```python
from build123d import *

# Parameters (mm, degrees)
SKETCH1_W           = 15
SKETCH1_H           = 15
SKETCH1_W_2         = 11
SKETCH1_H_2         = 11
BOSS_EXTRUDE1_DEPTH = 140
SKETCH2_R           = 1.6
CUT_EXTRUDE1_DEPTH  = 142.598022585
SKETCH3_R           = 1.6
CUT_EXTRUDE2_DEPTH  = 142.598022585


with BuildPart() as part:
    # Sketch1 → Boss-Extrude1 (new body)
    with BuildSketch(Plane(origin=(0, 0, 0), x_dir=(1, 0, 0), z_dir=(0, 1, 0))):
        with Locations((7.5, 7.5)):
            Rectangle(SKETCH1_W, SKETCH1_H)
        with Locations((7.5, 7.5)):
            Rectangle(SKETCH1_W_2, SKETCH1_H_2, mode=Mode.SUBTRACT)
    extrude(amount=BOSS_EXTRUDE1_DEPTH)

    # Sketch2 → Cut-Extrude1 (cut, through all)
    with BuildSketch(Plane(origin=(15, 0, 0), x_dir=(0, 0, -1), z_dir=(1, 0, 0))):
        with Locations((7.5, 13)):
            Circle(SKETCH2_R)
        with Locations((7.5, 37)):
            Circle(SKETCH2_R)
        with Locations((7.5, 103)):
            Circle(SKETCH2_R)
        with Locations((7.5, 127)):
            Circle(SKETCH2_R)
    extrude(amount=-CUT_EXTRUDE1_DEPTH, mode=Mode.SUBTRACT)

    # Sketch3 → Cut-Extrude2 (cut, through all)
    with BuildSketch(Plane.XY):
        with Locations((7.5, 85)):
            Circle(SKETCH3_R)
        with Locations((7.5, 55)):
            Circle(SKETCH3_R)
    extrude(amount=-CUT_EXTRUDE2_DEPTH, mode=Mode.SUBTRACT)


solid = part.part
```
Verification items for the finished model (mm, model axes). A direction names the side the tool comes from. Coordinates: 2 decimals unless noted, no trailing zeros. Loops run counter-clockwise (first coordinate to the right, second up) from the corner with the lowest first, then second, coordinate; pieces in that order, holes last. Notation, with made-up numbers: (30, 2) -> (44, 2) arc R26 ccw to (44, 25) -> close; hole circle Ø4 at (49.5, 73). An arc over 180 degrees is marked (long way). Answer in a Markdown table with one row per item. Add a question column.
1. Material ranges on probe 1 along Y at (x, z) = (7.5, -14.6); probe 2 along Y at (x, z) = (1.45, -7.5); probe 3 along X at (y, z) = (43, -4.25), recorded low to high. Write a range as [from, to].
2. Section check D-D, the plane y = 20. Enter the section's corners in (x, z).
3. Access from +Z, -Z, +X, -X, +Y, -Y to the whole of each face (thin tool, end or side, straight path). Record for faces 1 (the face through (13, 69, -7)), 2 (the face through (14, 0, -8)).
4. Section check B-B, the plane z = -11. Enter the section's corners in (x, y).
5. Draft check along X on faces 3 (the face through (14.01, 35.58, -8.24)), 4 (the face through (0, 69, -7)), 5 (the face through (5.9, 55.07, -0.99)), 6 (the face through (7.292, 86.586, -0.986)). Enter one of: +X half, -X half, draft (parallel to the pull), parting line (faces both ways), or undercut.
6. Section check A-A, the plane y = 103. Enter the section's corners in (x, z), then the cut area to 3 significant figures.
7. Section check C-C, the plane x = 7.5. Enter the section's corners in (y, z).
Derived:
| question | item | result |
|---|---|---|
| 1 | probe 1 | y = [0, 53.4], [56.6, 83.4], [86.6, 140] |
| 1 | probe 2 | y = [0, 11.4], [14.6, 35.4], [38.6, 101.4], [104.6, 125.4], [128.6, 140] |
| 1 | probe 3 | x = [0, 2], [13, 15] |
| 2 | outline | (0, -15) -> (15, -15) -> (15, 0) -> (0, 0) -> close; hole (2, -13) -> (13, -13) -> (13, -2) -> (2, -2) -> close |
| 3 | face 1 | +Y, -Y |
| 3 | face 2 | +Z, -Z, +X, -X, -Y |
| 4 | outline | (0, 0) -> (2, 0) -> (2, 140) -> (0, 140) -> close; (13, 0) -> (15, 0) -> (15, 140) -> (13, 140) -> close |
| 5 | face 3 | draft |
| 5 | face 4 | -X half |
| 5 | face 5 | undercut |
| 5 | face 6 | undercut |
| 6 | outline | (0, -15) -> (15, -15) -> (15, -9.1) -> (13, -9.1) -> (13, -13) -> (2, -13) -> (2, -9.1) -> (0, -9.1) -> close; (0, -5.9) -> (2, -5.9) -> (2, -2) -> (13, -2) -> (13, -5.9) -> (15, -5.9) -> (15, 0) -> (0, 0) -> close |
| 6 | area | 91.2 mm² |
| 7 | outline | (0, -15) -> (53.4, -15) -> (53.4, -13) -> (0, -13) -> close; (0, -2) -> (53.4, -2) -> (53.4, 0) -> (0, 0) -> close; (56.6, -15) -> (83.4, -15) -> (83.4, -13) -> (56.6, -13) -> close; (56.6, -2) -> (83.4, -2) -> (83.4, 0) -> (56.6, 0) -> close; (86.6, -15) -> (140, -15) -> (140, -13) -> (86.6, -13) -> close; (86.6, -2) -> (140, -2) -> (140, 0) -> (86.6, 0) -> close |
